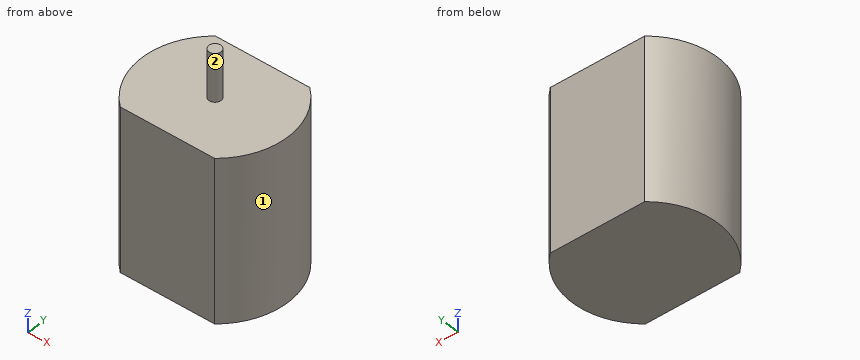
Autodesk Inventor part; units mm, degrees
ref_plane "YZ Plane" through (0, 0, 0) normal (1, 0, 0) x (0, 1, 0)
ref_plane "XZ Plane" through (0, 0, 0) normal (0, 1, 0) x (-1, 0, 0)
ref_plane "XY Plane" through (0, 0, 0) normal (0, 0, 1) x (1, 0, 0)
sketch "Sketch1" plane through (0, 0, 0) normal (0, 0, 1) x (1, 0, 0)
  line L0 (7.7639, -9.15) -> (-7.7639, -9.15)
  line L1 (-7.7639, -9.15) -> (-7.7639, 9.15) construction
  line L2 (-7.7639, 9.15) -> (7.7639, 9.15)
  line L3 (7.7639, -9.15) -> (-7.7639, 9.15) construction
  line L4 (-7.7639, -9.15) -> (7.7639, 9.15) construction
  arc A0 (-7.7639, 9.15) -> (-7.7639, -9.15) centre (0, 0) ccw
  arc A1 (7.7639, -9.15) -> (7.7639, 9.15) centre (0, 0) ccw
  dimension "d8" = 18.3
extrude "Extrusion1" add sketch "Sketch1" along normal blind 26.9
sketch "Sketch2" plane through (0, 0, 26.9) normal (0, 0, 1) x (1, 0, 0)
  circle A0 centre (0, 0) radius 1
  dimension "d4" = 2
extrude "Extrusion2" add sketch "Sketch2" along normal blind 7.9
properties part number "dc_motor"
Could you check a few things on this model? Use its own coordinates, in mm. Face numbers are marked on the shaded views. A direction names the side the tool comes from. Round coordinates to 2 decimals unless told otherwise and drop trailing zeros. Write each loop counter-clockwise with the first axis right and the second up, starting at its lowest first coordinate (ties: lowest second). Pieces come first, ordered by that corner, then holes. Notation, with made-up numbers: M 28,38.25 L 58,38.25 A23 ccw 58,72.25 Z; hole C 5.25,52.5 d11. An arc over 180 degrees is marked long. Write each question's results on one line, items separated by ' | '. Start each with the question number.
1. Imagine slicing it at C-C on z = 5.5. List the corners of the cut face in (x, y) for me, and give its area (3 significant figures).
2. Imagine slicing it at B-B on y = 0. List the corners of the cut face in (x, z) for me.
3. I need wall thicknesses on L1, parallel to Z at x = 5.75, y = 8.25; L2, parallel to X at y = 7.75, z = 2; L3, parallel to Y at x = -0.5, z = 32. Which ranges of each line are inside material? Lowest first, please. Write a range as from..to.
4. On a 3-axis mill with a long thin cutter (end or side, diameter ignored), from which of +Z, -Z, +X, -X, +Y, -Y can I reach the whole of each face in a straight line? I mean the marked faces 1 and 2. Say none if no direction works.
5. Imagine slicing it at A-A on x = 0. List the corners of the cut face in (y, z) for me, and give its area (3 significant figures).
6. Imagine slicing it at D-D on y = 5. List the corners of the cut face in (x, z) for me, and give its area (3 significant figures).
Result sheet:
1) outline: M -7.76,-9.15 L 7.76,-9.15 A12 ccw 7.76,9.15 L -7.76,9.15 A12 ccw Z | area: 392 mm^2
2) outline: M -12,0 L 12,0 L 12,26.9 L 1,26.9 L 1,34.8 L -1,34.8 L -1,26.9 L -12,26.9 Z
3) L1: z = 0..26.9 | L2: x = -9.16..9.16 | L3: y = -0.87..0.87
4) face 1: +Z, -Z, +X | face 2: +Z
5) outline: M -9.15,0 L 9.15,0 L 9.15,26.9 L 1,26.9 L 1,34.8 L -1,34.8 L -1,26.9 L -9.15,26.9 Z | area: 508 mm^2
6) outline: M -10.91,0 L 10.91,0 L 10.91,26.9 L -10.91,26.9 Z | area: 587 mm^2
